```python
from build123d import *

# Parameters (mm, degrees)
CUT_EXTRUDE1_DEPTH       = 0.84455
CUT_EXTRUDE1_DEPTH_BACK  = 0.84455
BOSS_EXTRUDE1_DEPTH      = 0.79375
BOSS_EXTRUDE1_DEPTH_BACK = 0.79375


with BuildPart() as part:
    # Sketch1 → Revolve1 (revolve)
    with BuildSketch(Plane(origin=(0, 0, 0), x_dir=(0, 0, -1), z_dir=(1, 0, 0))):
        Polygon((-44.323, 0), (-44.323, 4.3815), (-43.942, 4.7625), (17.018, 4.7625), (17.399, 4.3815), (17.399, 0), align=None)
    revolve(axis=Axis((0, 0, -17.399), (0, 0, 1)))

    # Sketch2 → Cut-Extrude1 (cut, two sides)
    with BuildSketch(Plane(origin=(0, 0, 0), x_dir=(0, 0, -1), z_dir=(1, 0, 0))) as cut_extrude1_sk:
        with BuildLine():
            Line((-25.3873, 5.5753), (-37.8587, 5.5753))
            ThreePointArc((-37.8587, 5.5753), (-31.623, 0.424693809), (-25.3873, 5.5753))
        make_face()
    extrude(amount=CUT_EXTRUDE1_DEPTH, mode=Mode.SUBTRACT)
    extrude(cut_extrude1_sk.sketch, amount=-CUT_EXTRUDE1_DEPTH_BACK, mode=Mode.SUBTRACT)

    # Sketch3 → Boss-Extrude1 (add, two sides)
    with BuildSketch(Plane(origin=(0, 0, 0), x_dir=(0, 0, -1), z_dir=(1, 0, 0))) as boss_extrude1_sk:
        with BuildLine():
            Line((-31.75, 0.425963936), (-31.75, 0.169400396))
            Line((-31.75, 0.169400396), (-31.496, 0.169400396))
            Line((-31.496, 0.169400396), (-31.496, 0.425963936))
            ThreePointArc((-31.496, 0.425963936), (-27.530335428, 1.919531948), (-25.3873, 5.5753))
            Line((-25.3873, 5.5753), (-37.8587, 5.5753))
            ThreePointArc((-37.8587, 5.5753), (-35.715664572, 1.919531948), (-31.75, 0.425963936))
        make_face()
    extrude(amount=BOSS_EXTRUDE1_DEPTH)
    extrude(boss_extrude1_sk.sketch, amount=-BOSS_EXTRUDE1_DEPTH_BACK)


solid = part.part
```
Verification items for the finished model (mm, model axes). A direction names the side the tool comes from. Give positions to 0.01 mm unless a question says otherwise; leave off trailing zeros. Loops run counter-clockwise (first coordinate to the right, second up) from the corner with the lowest first, then second, coordinate; pieces in that order, holes last.
1. Section check D-D, the plane z = 18. Enter the section's corners in (x, y) (1 decimal).
2. Section check A-A, the plane x = 0. Enter the section's corners in (y, z).
3. Mould release check, pull along Z, two halves, no side actions. Record for faces 1 (the flat face through (0, 0, 44.323)), 2 (the flat face through (-0.794, 5, 32)), 3 (the cylindrical face through (2.9, -3.78, 13.04)): released by +Z, released by -Z, zero draft, split by the parting line, or undercut.
4. Set-up check for faces 4 (the flat face through (0.794, 5, 32)), 5 (the flat face through (0, 5.575, 32)): record each of +Z, -Z, +X, -X, +Y, -Y from which the full face is reachable in a straight line by a thin tool's end or side.
5. Thickness scan on line 1 (Y direction, x = 0, z = 2); line 2 (X direction, y = -3.75, z = 33); line 3 (Y direction, x = -1.75, z = -8.5). Record the ranges inside material, lowest first.
6. Section check C-C, the plane y = 3.25. Count the separate pieces of the cut face and the enclosed holes in it, then the cut area to 3 significant figures.
7. Go/stop test with flat-tipped pins: pin 1 Ø3.5 at (y, z) = (2, 32.5) entering from -X; pin 2 Ø4 at (y, z) = (3.5, 17) entering from +X; pin 3 Ø2.5 at (y, z) = (3, 34) entering from +X; pin 4 Ø2 at (y, z) = (0.5, 7) entering from +X. Record where each tip stops, or that it passes through.
Geometry says:
1. outline: circle Ø9.5 at (0, 0)
2. outline: (-4.76, -17.02) - (-4.38, -17.4) - (4.38, -17.4) - (4.76, -17.02) - (4.76, 25.6) arc R6.35 ccw to (5.58, 25.39) - (5.58, 37.86) arc R6.35 ccw to (4.76, 37.65) - (4.76, 43.94) - (4.38, 44.32) - (-4.38, 44.32) - (-4.76, 43.94) - close
3. face 1: released by +Z
3. face 2: undercut
3. face 3: zero draft
4. face 4: +Y
4. face 5: +Z, -Z, +X, -X, +Y
5. line 1: y = -4.76 to 4.76
5. line 2: x = -2.94 to 2.94
5. line 3: y = -4.43 to 4.43
6. separate pieces: 1
6. enclosed holes: 2
6. area: 428 mm2
7. pin 1: stops at x = -4.76
7. pin 2: stops at x = 4.52
7. pin 3: stops at x = 4.43
7. pin 4: stops at x = 4.76
